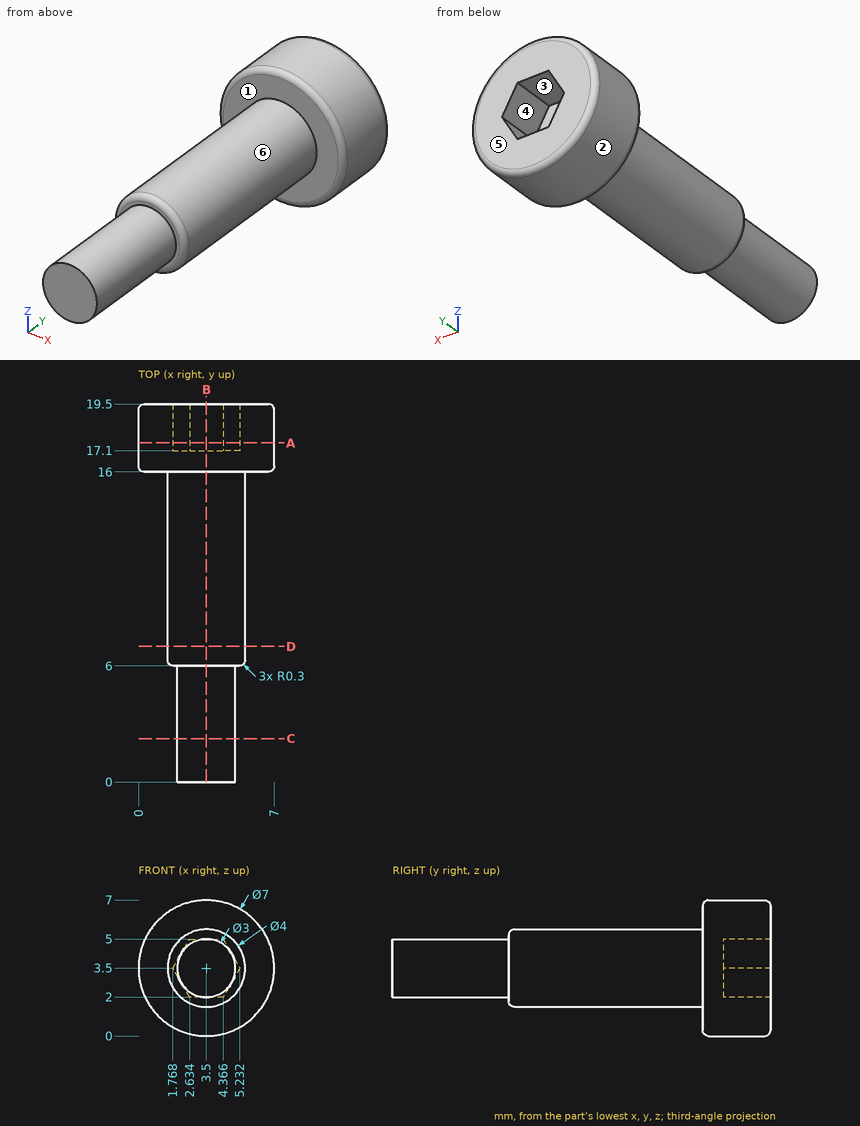
Could you check a few things on this drawing? It's one solid part, dimensions in mm from its lowest x, y, z. A direction names the side the tool comes from. Coordinates: 2 decimals unless noted, no trailing zeros. Order: outer loops, then holes, each group sorted by start corner. A loop starts at its lowest first (then second) coordinate and runs counter-clockwise, first axis right, second up. Notation, with made-up numbers: (-1, 13.5) -> (52, 13.5) arc R28 ccw to (52, 34.5) -> close; hole circle Ø7 at (72, 74). An arc over 180 degrees is marked (long way). One line per item, written item: value. Start each with the question number.
1) Imagine slicing it at D-D on y = 7. List the corners of the cut face in (x, z) for me, plus the area to 3 significant figures.
2) If I drill on L1, parallel to X at y = 14, z = 4.5; L2, parallel to Z at x = 4.75, y = 18.75 (1 decimal); L3, parallel to Y at x = 3.5, z = 0.75, over which ranges is the centre line in solid material (lowest first)? Write a range as [from, to].
3) We'd pull the mould along X, two halves only. Please class the marked faces 1, 2 and 3: +X half, -X half, draft (parallel to the pull), parting line (faces both ways), or undercut.
4) Which directions (+Z, -Z, +X, -X, +Y, -Y) give clear straight access to the entire face, cutting with the end or side of a thin tool? Please do the marked faces 4, 5 and 6.
5) Imagine slicing it at A-A on y = 17.5. List the corners of the cut face in (x, z) for me, plus the area to 3 significant figures.
6) Imagine slicing it at C-C on y = 2.25. List the corners of the cut face in (x, z) for me, plus the area to 3 significant figures.
7) Imagine slicing it at B-B on x = 3.5. List the corners of the cut face in (y, z) for me, plus the area to 3 significant figures.
8) I'm going to push flat-ended pins straight in: pin 1 (1 mm diameter, centred on y = 12.5, z = 2, fed in from +X); pin 2 (0.9 mm diameter, centred on x = 3.5, z = 4, fed in from +Y); pin 3 (1.5 mm diameter, centred on x = 2, y = 5.5, fed in from -Z). Where does each tip first touch, or does it pass through?
Answer list:
1. outline: circle Ø4 at (3.5, 3.5)
1. area: 12.6 mm2
2. L1: x = [1.77, 5.23]
2. L2: z = [0.2, 2.7], [4.3, 6.8]
2. L3: y = [16, 19.5]
3. face 1: draft
3. face 2: parting line
3. face 3: undercut
4. face 4: +Y
4. face 5: +Z, -Z, +X, -X, +Y
4. face 6: -Y
5. outline: circle Ø7 at (3.5, 3.5); hole (1.77, 3.5) -> (2.63, 2) -> (4.37, 2) -> (5.23, 3.5) -> (4.37, 5) -> (2.63, 5) -> close
5. area: 30.7 mm2
6. outline: circle Ø3 at (3.5, 3.5)
6. area: 7.07 mm2
7. outline: (0, 2) -> (6, 2) -> (6, 1.8) arc R0.3 ccw to (6.3, 1.5) -> (16, 1.5) -> (16, 0.3) arc R0.3 ccw to (16.3, 0) -> (19.2, 0) arc R0.3 ccw to (19.5, 0.3) -> (19.5, 2) -> (17.1, 2) -> (17.1, 5) -> (19.5, 5) -> (19.5, 6.7) arc R0.3 ccw to (19.2, 7) -> (16.3, 7) arc R0.3 ccw to (16, 6.7) -> (16, 5.5) -> (6.3, 5.5) arc R0.3 ccw to (6, 5.2) -> (6, 5) -> (0, 5) -> close
7. area: 75.2 mm2
8. pin 1: stops at x = 5.23
8. pin 2: stops at y = 17.1
8. pin 3: stops at z = 1.89
